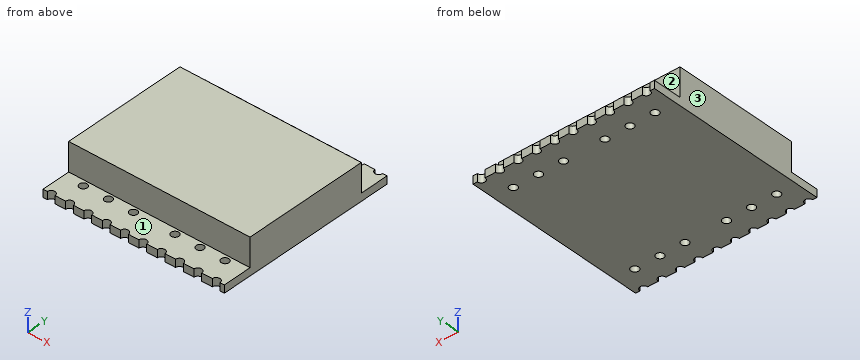
```python
from build123d import *

# Parameters (mm, degrees)
SKETCH_1_W                    = 18.8
SKETCH_1_H                    = 19
EXTRUDE_1_DEPTH               = 0.8
SKETCH_2_W                    = 18.8
SKETCH_2_H                    = 13
EXTRUDE_2_DEPTH               = 2.95
CUT_EXTRUDE_1_DEPTH           = 14.686215693
PATTERN_LINEAR_1_COUNT        = 10
PATTERN_LINEAR_1_PITCH        = 1.9
PATTERN_LINEAR_1_COPY_1_DEPTH = 14.686215693
PATTERN_LINEAR_1_COPY_2_DEPTH = 14.686215693
PATTERN_LINEAR_1_COPY_3_DEPTH = 14.686215693
PATTERN_LINEAR_1_COPY_4_DEPTH = 14.686215693
PATTERN_LINEAR_1_COPY_5_DEPTH = 14.686215693
PATTERN_LINEAR_1_COPY_6_DEPTH = 14.686215693
PATTERN_LINEAR_1_COPY_7_DEPTH = 14.686215693
PATTERN_LINEAR_1_COPY_8_DEPTH = 14.686215693
PATTERN_LINEAR_1_COPY_9_DEPTH = 14.686215693
SKETCH_4_R                    = 0.4
CUT_EXTRUDE_2_DEPTH           = 14.686215693
PATTERN_LINEAR_2_COUNT        = 3
PATTERN_LINEAR_2_PITCH        = 2.6
MIRROR_2_COPY_1_SKETCH_R      = 0.4
MIRROR_2_COPY_1_DEPTH         = 14.686215693
MIRROR_2_COPY_2_SKETCH_R      = 0.4
MIRROR_2_COPY_2_DEPTH         = 14.686215693
MIRROR_3_COPY_1_SKETCH_R      = 0.4
MIRROR_3_COPY_1_DEPTH         = 14.686215693
MIRROR_3_COPY_2_SKETCH_R      = 0.4
MIRROR_3_COPY_2_DEPTH         = 14.686215693
MIRROR_3_COPY_3_SKETCH_R      = 0.4
MIRROR_3_COPY_3_DEPTH         = 14.686215693
MIRROR_3_COPY_4_SKETCH_R      = 0.4
MIRROR_3_COPY_4_DEPTH         = 14.686215693
MIRROR_3_COPY_5_SKETCH_R      = 0.4
MIRROR_3_COPY_5_DEPTH         = 14.686215693


with BuildPart() as part:
    # Эскиз1 → Бобышка-Вытянуть1 (new body)
    with BuildSketch(Plane.XY):
        Rectangle(SKETCH_1_W, SKETCH_1_H)
    extrude(amount=EXTRUDE_1_DEPTH)

    # Эскиз2 → Бобышка-Вытянуть2 (add)
    with BuildSketch(Plane.XY.offset(0.8)):
        Rectangle(SKETCH_2_W, SKETCH_2_H)
    extrude(amount=EXTRUDE_2_DEPTH)

    # Эскиз3 → Вырез-Вытянуть1 (cut, symmetric)
    with BuildSketch(Plane.XY.offset(0.8)):
        with BuildLine():
            Line((-8.95, -9.5), (-8.15, -9.5))
            ThreePointArc((-8.15, -9.5), (-8.55, -9.1), (-8.95, -9.5))
        make_face()
    cut_extrude_1 = extrude(amount=CUT_EXTRUDE_1_DEPTH, both=True, mode=Mode.SUBTRACT)

    # Зеркальное отражение1: Вырез-Вытянуть1 across plane
    add(cut_extrude_1.mirror(Plane.ZX), mode=Mode.SUBTRACT)

    # Линейный массив1: Вырез-Вытянуть1 ×10
    with Locations(*[(i * PATTERN_LINEAR_1_PITCH, 0, 0) for i in range(1, PATTERN_LINEAR_1_COUNT)]):
        add(cut_extrude_1, mode=Mode.SUBTRACT)

    # Линейный массив1 copy 1 sketch → Линейный массив1 copy 1 (cut, symmetric)
    with BuildSketch(Plane(origin=(1.9, 0, 0.8), x_dir=(1, 0, 0), z_dir=(0, 0, 1))):
        with BuildLine():
            Line((-8.95, 9.5), (-8.15, 9.5))
            ThreePointArc((-8.15, 9.5), (-8.55, 9.1), (-8.95, 9.5))
        make_face()
    extrude(amount=PATTERN_LINEAR_1_COPY_1_DEPTH, both=True, mode=Mode.SUBTRACT)

    # Линейный массив1 copy 2 sketch → Линейный массив1 copy 2 (cut, symmetric)
    with BuildSketch(Plane(origin=(3.8, 0, 0.8), x_dir=(1, 0, 0), z_dir=(0, 0, 1))):
        with BuildLine():
            Line((-8.95, 9.5), (-8.15, 9.5))
            ThreePointArc((-8.15, 9.5), (-8.55, 9.1), (-8.95, 9.5))
        make_face()
    extrude(amount=PATTERN_LINEAR_1_COPY_2_DEPTH, both=True, mode=Mode.SUBTRACT)

    # Линейный массив1 copy 3 sketch → Линейный массив1 copy 3 (cut, symmetric)
    with BuildSketch(Plane(origin=(5.7, 0, 0.8), x_dir=(1, 0, 0), z_dir=(0, 0, 1))):
        with BuildLine():
            Line((-8.95, 9.5), (-8.15, 9.5))
            ThreePointArc((-8.15, 9.5), (-8.55, 9.1), (-8.95, 9.5))
        make_face()
    extrude(amount=PATTERN_LINEAR_1_COPY_3_DEPTH, both=True, mode=Mode.SUBTRACT)

    # Линейный массив1 copy 4 sketch → Линейный массив1 copy 4 (cut, symmetric)
    with BuildSketch(Plane(origin=(7.6, 0, 0.8), x_dir=(1, 0, 0), z_dir=(0, 0, 1))):
        with BuildLine():
            Line((-8.95, 9.5), (-8.15, 9.5))
            ThreePointArc((-8.15, 9.5), (-8.55, 9.1), (-8.95, 9.5))
        make_face()
    extrude(amount=PATTERN_LINEAR_1_COPY_4_DEPTH, both=True, mode=Mode.SUBTRACT)

    # Линейный массив1 copy 5 sketch → Линейный массив1 copy 5 (cut, symmetric)
    with BuildSketch(Plane(origin=(9.5, 0, 0.8), x_dir=(1, 0, 0), z_dir=(0, 0, 1))):
        with BuildLine():
            Line((-8.95, 9.5), (-8.15, 9.5))
            ThreePointArc((-8.15, 9.5), (-8.55, 9.1), (-8.95, 9.5))
        make_face()
    extrude(amount=PATTERN_LINEAR_1_COPY_5_DEPTH, both=True, mode=Mode.SUBTRACT)

    # Линейный массив1 copy 6 sketch → Линейный массив1 copy 6 (cut, symmetric)
    with BuildSketch(Plane(origin=(11.4, 0, 0.8), x_dir=(1, 0, 0), z_dir=(0, 0, 1))):
        with BuildLine():
            Line((-8.95, 9.5), (-8.15, 9.5))
            ThreePointArc((-8.15, 9.5), (-8.55, 9.1), (-8.95, 9.5))
        make_face()
    extrude(amount=PATTERN_LINEAR_1_COPY_6_DEPTH, both=True, mode=Mode.SUBTRACT)

    # Линейный массив1 copy 7 sketch → Линейный массив1 copy 7 (cut, symmetric)
    with BuildSketch(Plane(origin=(13.3, 0, 0.8), x_dir=(1, 0, 0), z_dir=(0, 0, 1))):
        with BuildLine():
            Line((-8.95, 9.5), (-8.15, 9.5))
            ThreePointArc((-8.15, 9.5), (-8.55, 9.1), (-8.95, 9.5))
        make_face()
    extrude(amount=PATTERN_LINEAR_1_COPY_7_DEPTH, both=True, mode=Mode.SUBTRACT)

    # Линейный массив1 copy 8 sketch → Линейный массив1 copy 8 (cut, symmetric)
    with BuildSketch(Plane(origin=(15.2, 0, 0.8), x_dir=(1, 0, 0), z_dir=(0, 0, 1))):
        with BuildLine():
            Line((-8.95, 9.5), (-8.15, 9.5))
            ThreePointArc((-8.15, 9.5), (-8.55, 9.1), (-8.95, 9.5))
        make_face()
    extrude(amount=PATTERN_LINEAR_1_COPY_8_DEPTH, both=True, mode=Mode.SUBTRACT)

    # Линейный массив1 copy 9 sketch → Линейный массив1 copy 9 (cut, symmetric)
    with BuildSketch(Plane(origin=(17.1, 0, 0.8), x_dir=(1, 0, 0), z_dir=(0, 0, 1))):
        with BuildLine():
            Line((-8.95, 9.5), (-8.15, 9.5))
            ThreePointArc((-8.15, 9.5), (-8.55, 9.1), (-8.95, 9.5))
        make_face()
    extrude(amount=PATTERN_LINEAR_1_COPY_9_DEPTH, both=True, mode=Mode.SUBTRACT)

    # Эскиз4 → Вырез-Вытянуть2 (cut, symmetric)
    with BuildSketch(Plane.XY.offset(0.8)):
        with Locations((-2.15, -7.1)):
            Circle(SKETCH_4_R)
    cut_extrude_2 = extrude(amount=CUT_EXTRUDE_2_DEPTH, both=True, mode=Mode.SUBTRACT)

    # Линейный массив2: Вырез-Вытянуть2 ×3
    with Locations(*[(-i * PATTERN_LINEAR_2_PITCH, 0, 0) for i in range(1, PATTERN_LINEAR_2_COUNT)]):
        add(cut_extrude_2, mode=Mode.SUBTRACT)

    # Зеркальное отражение2: Вырез-Вытянуть2 across plane
    add(cut_extrude_2.mirror(Plane.ZX), mode=Mode.SUBTRACT)

    # Зеркальное отражение2 copy 1 sketch → Зеркальное отражение2 copy 1 (cut, symmetric)
    with BuildSketch(Plane(origin=(-2.6, 0, 0.8), x_dir=(1, 0, 0), z_dir=(0, 0, 1))):
        with Locations((-2.15, 7.1)):
            Circle(MIRROR_2_COPY_1_SKETCH_R)
    extrude(amount=MIRROR_2_COPY_1_DEPTH, both=True, mode=Mode.SUBTRACT)

    # Зеркальное отражение2 copy 2 sketch → Зеркальное отражение2 copy 2 (cut, symmetric)
    with BuildSketch(Plane(origin=(-5.2, 0, 0.8), x_dir=(1, 0, 0), z_dir=(0, 0, 1))):
        with Locations((-2.15, 7.1)):
            Circle(MIRROR_2_COPY_2_SKETCH_R)
    extrude(amount=MIRROR_2_COPY_2_DEPTH, both=True, mode=Mode.SUBTRACT)

    # Зеркальное отражение3: Вырез-Вытянуть2 across plane
    add(cut_extrude_2.mirror(Plane(origin=(0, 0, 0), x_dir=(0, 0, 1), z_dir=(1, 0, 0))), mode=Mode.SUBTRACT)

    # Зеркальное отражение3 copy 1 sketch → Зеркальное отражение3 copy 1 (cut, symmetric)
    with BuildSketch(Plane(origin=(2.6, 0, 0.8), x_dir=(-1, 0, 0), z_dir=(0, 0, 1))):
        with Locations((-2.15, 7.1)):
            Circle(MIRROR_3_COPY_1_SKETCH_R)
    extrude(amount=MIRROR_3_COPY_1_DEPTH, both=True, mode=Mode.SUBTRACT)

    # Зеркальное отражение3 copy 2 sketch → Зеркальное отражение3 copy 2 (cut, symmetric)
    with BuildSketch(Plane(origin=(5.2, 0, 0.8), x_dir=(-1, 0, 0), z_dir=(0, 0, 1))):
        with Locations((-2.15, 7.1)):
            Circle(MIRROR_3_COPY_2_SKETCH_R)
    extrude(amount=MIRROR_3_COPY_2_DEPTH, both=True, mode=Mode.SUBTRACT)

    # Зеркальное отражение3 copy 3 sketch → Зеркальное отражение3 copy 3 (cut, symmetric)
    with BuildSketch(Plane(origin=(0, 0, 0.8), x_dir=(-1, 0, 0), z_dir=(0, 0, 1))):
        with Locations((-2.15, -7.1)):
            Circle(MIRROR_3_COPY_3_SKETCH_R)
    extrude(amount=MIRROR_3_COPY_3_DEPTH, both=True, mode=Mode.SUBTRACT)

    # Зеркальное отражение3 copy 4 sketch → Зеркальное отражение3 copy 4 (cut, symmetric)
    with BuildSketch(Plane(origin=(2.6, 0, 0.8), x_dir=(-1, 0, 0), z_dir=(0, 0, 1))):
        with Locations((-2.15, -7.1)):
            Circle(MIRROR_3_COPY_4_SKETCH_R)
    extrude(amount=MIRROR_3_COPY_4_DEPTH, both=True, mode=Mode.SUBTRACT)

    # Зеркальное отражение3 copy 5 sketch → Зеркальное отражение3 copy 5 (cut, symmetric)
    with BuildSketch(Plane(origin=(5.2, 0, 0.8), x_dir=(-1, 0, 0), z_dir=(0, 0, 1))):
        with Locations((-2.15, -7.1)):
            Circle(MIRROR_3_COPY_5_SKETCH_R)
    extrude(amount=MIRROR_3_COPY_5_DEPTH, both=True, mode=Mode.SUBTRACT)


solid = part.part
```
Work out the finished part from the listing and answer in its coordinate system (mm). Face numbers are marked on the shaded views. A direction names the side the tool comes from. Give positions to 0.01 mm unless a question says otherwise; leave off trailing zeros. Order: outer loops, then holes, each group sorted by start corner. A loop starts at its lowest first (then second) coordinate and runs counter-clockwise, first axis right, second up. Notation, with made-up numbers: (48.25, 39) - (88.25, 39) arc R21 ccw to (88.25, 69) - close; hole circle Ø7 at (12, 76.25). An arc over 180 degrees is marked (long way). One line per item, written item: value. Start each with the question number.
1. Which of the six approach directions +Z, -Z, +X, -X, +Y, -Y give full straight-line access (tool end or side, diameter ignored) to the marked faces 1, 2 and 3?
2. Section C-C, the plane x = -4.75 is taken. Write down the section's boundary in (y, z).
3. Section D-D, the plane z = 1.8 is taken. Write down the section's boundary in (x, y), then the cut area to 3 significant figures.
4. Section B-B, the plane z = 0.5 is taken. Count the separate pieces of the cut face and the enclosed holes in it, then the cut area to 3 significant figures.
5. Each of these flat-tipped pins is pushed along its axis until it touches: pin 1 Ø0.9 at (x, y) = (3, -8) entering from +Z; pin 2 Ø1 at (x, z) = (-7, 2.5) entering from -Y; pin 3 Ø0.9 at (x, z) = (3.5, 3) entering from +Y. Where does it stop, or does it pass through?
6. Consider line 1 (Y direction, x = -4.75, z = 0.2); line 2 (Y direction, x = 7.35, z = 0.3); line 3 (Z direction, x = -5, y = 7.5). Determine where each line is inside the solid, lowest interval first.
7. Section A-A, the plane x = -2.15 is taken. Write down the section's boundary in (y, z), then the cut area to 3 significant figures.
Filled sheet:
1. face 1: +Z, +X, -X, -Y
1. face 2: +Z, +X, -X, +Y
1. face 3: +Z, -Z, -X, +Y, -Y
2. outline: (-9.1, 0) - (-7.5, 0) - (-7.5, 0.8) - (-9.1, 0.8) - close; (-6.7, 0) - (6.7, 0) - (6.7, 0.8) - (6.5, 0.8) - (6.5, 3.75) - (-6.5, 3.75) - (-6.5, 0.8) - (-6.7, 0.8) - close; (7.5, 0) - (9.1, 0) - (9.1, 0.8) - (7.5, 0.8) - close
3. outline: (-9.4, -6.5) - (9.4, -6.5) - (9.4, 6.5) - (-9.4, 6.5) - close
3. area: 244 mm²
4. separate pieces: 1
4. enclosed holes: 12
4. area: 346 mm²
5. pin 1: z = 0.8
5. pin 2: y = -6.5
5. pin 3: y = 6.5
6. line 1: -9.1 to -7.5, -6.7 to 6.7, 7.5 to 9.1
6. line 2: -9.5 to -7.5, -6.7 to 6.7, 7.5 to 9.5
6. line 3: 0 to 0.8
7. outline: (-9.5, 0) - (-7.5, 0) - (-7.5, 0.8) - (-9.5, 0.8) - close; (-6.7, 0) - (6.7, 0) - (6.7, 0.8) - (6.5, 0.8) - (6.5, 3.75) - (-6.5, 3.75) - (-6.5, 0.8) - (-6.7, 0.8) - close; (7.5, 0) - (9.5, 0) - (9.5, 0.8) - (7.5, 0.8) - close
7. area: 52.3 mm²
